Study the drawing (mm; zero at the part's minimum x, y, z) and answer. Give positions to 0.01 mm unless a question says otherwise; leave off trailing zeros. Write each loop counter-clockwise with the first axis right and the second up, starting at its lowest first coordinate (ties: lowest second). Pieces come first, ordered by that corner, then holes. Notation, with made-up numbers: (15.25, 24.25) - (40.25, 24.25) arc R32 ccw to (40.25, 61.25) - close; hole circle Ø7 at (18, -26.75). An arc over 180 degrees is marked (long way). Write each question's results on one line, items separated by ' | '. Start each with the question number.
Q1. Section A-A (x = 14.2) is taken. Determine the outline of the cut face in (y, z).
Q2. Flat-ended cylindrical pins translate along their axes: pin 1 Ø4 at (x, z) = (17.5, 29.5) entering from +Y; pin 2 Ø10 at (y, z) = (24.5, 43) entering from +X; pin 3 Ø8 at (x, y) = (9.5, 21.5) entering from +Z. Find the tip coordinate at first contact, or state that the pin passes through.
Q3. Section D-D (x = 5.7) is taken. Determine the outline of the cut face in (y, z) (1 decimal).
Q4. Find the intervals of material crossed by probe 1 along Z at (x, y) = (2.5, 17.5); probe 2 along Y at (x, z) = (5.7, 56.9) (1 decimal); probe 3 along X at (y, z) = (12, 23), in increasing order.
Q5. Section C-C (z = 45) is taken. Determine the outline of the cut face in (x, y).
Q6. Section B-B (y = 14.2) is taken. Determine the outline of the cut face in (x, z).
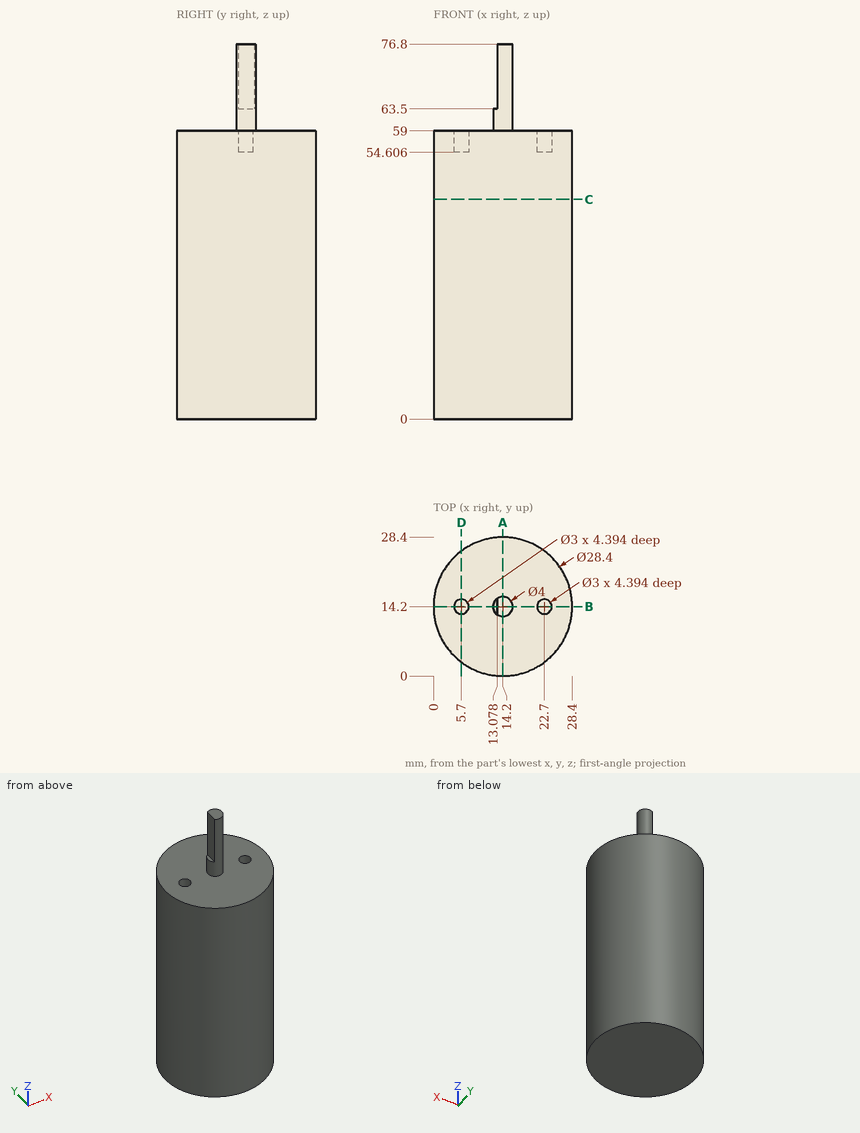
Answers below:
1) outline: (0, 0) - (28.4, 0) - (28.4, 59) - (16.2, 59) - (16.2, 76.8) - (12.2, 76.8) - (12.2, 59) - (0, 59) - close
2) pin 1: stops at y = 28.34 | pin 2: stops at x = 27.37 | pin 3: stops at z = 59
3) outline: (2.8, 0) - (25.6, 0) - (25.6, 59) - (15.7, 59) - (15.7, 54.6) - (12.7, 54.6) - (12.7, 59) - (2.8, 59) - close
4) probe 1: z = 0 to 59 | probe 2: y = 2.8 to 12.7, 15.7 to 25.6 | probe 3: x = 0.17 to 28.23
5) outline: circle Ø28.4 at (14.2, 14.2)
6) outline: (0, 0) - (28.4, 0) - (28.4, 59) - (24.2, 59) - (24.2, 54.61) - (21.2, 54.61) - (21.2, 59) - (16.2, 59) - (16.2, 76.8) - (13.08, 76.8) - (13.08, 63.5) - (12.2, 63.5) - (12.2, 59) - (7.2, 59) - (7.2, 54.61) - (4.2, 54.61) - (4.2, 59) - (0, 59) - close
